from build123d import *

# Parameters (mm, degrees)
SKETCH1_W           = 51
SKETCH1_H           = 51
SKETCH1_R           = 1.5
BOSS_EXTRUDE1_DEPTH = 3


with BuildPart() as part:
    # Sketch1 → Boss-Extrude1 (new body)
    with BuildSketch(Plane(origin=(0, 0, 0), x_dir=(1, 0, 0), z_dir=(0, 1, 0))):
        Polygon((85, 1.25), (85, 3.5), (28, 3.5), (28, 28), (3.5, 28), (3.5, 85), (1.25, 85), (1.25, 100), (-1.25, 100), (-1.25, 85), (-3.5, 85), (-3.5, 28), (-28, 28), (-28, 3.5), (-85, 3.5), (-85, 1.25), (-100, 1.25), (-100, -1.25), (-85, -1.25), (-85, -3.5), (-28, -3.5), (-28, -28), (-3.5, -28), (-3.5, -85), (-1.25, -85), (-1.25, -100), (1.25, -100), (1.25, -85), (3.5, -85), (3.5, -28), (28, -28), (28, -3.5), (85, -3.5), (85, -1.25), (100, -1.25), (100, 1.25), align=None)
        Rectangle(SKETCH1_W, SKETCH1_H, mode=Mode.SUBTRACT)
        with Locations(Location((36, 0, 0), (0, 0, 270))):
            Circle(SKETCH1_R, mode=Mode.SUBTRACT)
        with Locations(Location((77, 0, 0), (0, 0, 270))):
            Circle(SKETCH1_R, mode=Mode.SUBTRACT)
        with Locations(Location((0, 77, 0), (0, 0, 270))):
            Circle(SKETCH1_R, mode=Mode.SUBTRACT)
        with Locations(Location((0, 36, 0), (0, 0, 270))):
            Circle(SKETCH1_R, mode=Mode.SUBTRACT)
        with Locations(Location((0, -36, 0), (0, 0, 270))):
            Circle(SKETCH1_R, mode=Mode.SUBTRACT)
        with Locations(Location((0, -77, 0), (0, 0, 270))):
            Circle(SKETCH1_R, mode=Mode.SUBTRACT)
        with Locations(Location((-36, 0, 0), (0, 0, 270))):
            Circle(SKETCH1_R, mode=Mode.SUBTRACT)
        with Locations(Location((-77, 0, 0), (0, 0, 270))):
            Circle(SKETCH1_R, mode=Mode.SUBTRACT)
    extrude(amount=BOSS_EXTRUDE1_DEPTH)


solid = part.part
Geometry: final body of the model. Coordinates: model frame, mm. Round coordinates to 2 decimals unless told otherwise and drop trailing zeros. Order: outer loops, then holes, each group sorted by start corner. A loop starts at its lowest first (then second) coordinate and runs counter-clockwise, first axis right, second up. Notation, with made-up numbers: (22.5, 8.5) -> (34.5, 8.5) arc R10 ccw to (34.5, 14.5) -> close; hole circle Ø2 at (-24.5, 60.5). An arc over 180 degrees is marked (long way). Put each result on its own line as item: value. Start each with the question number.
Q1. Section B-B on x = -49. Return the cut outline in (y, z).
Q2. Section A-A on x = -8. Return the cut outline in (y, z).
Q3. Section C-C on y = 1.85. Give the number of separate pieces and of enclosed holes in the cut face, and give its area (3 significant figures).
Q4. Line query: probe 1 along X at (y, z) = (1.7, 0); probe 2 along X at (y, z) = (1.9, -9.5); probe 3 along X at (y, z) = (1.5, 77). Output: solid intervals per line, ascending.
Q5. Section D-D on z = 32. Return the cut outline in (x, y), and give its area (3 significant figures).
Q6. First-contact query: pin 1 (2.5 mm diameter, centred on x = 0, z = -36, fed in from +Y); pin 2 (1 mm diameter, centred on x = -21, y = 2.5, fed in from +Z); pin 3 (1.1 mm diameter, centred on y = 2, z = -2.5, fed in from +X); pin 4 (1.5 mm diameter, centred on x = -59, y = 1, fed in from +Z). Flat tips, straight axial feed; report the tip coordinate or a pass-through.
Ans:
1. outline: (0, -3.5) -> (3, -3.5) -> (3, 3.5) -> (0, 3.5) -> close
2. outline: (0, -28) -> (3, -28) -> (3, -25.5) -> (0, -25.5) -> close; (0, 25.5) -> (3, 25.5) -> (3, 28) -> (0, 28) -> close
3. separate pieces: 1
3. enclosed holes: 9
3. area: 2,220 mm2
4. probe 1: x = -100 to -78.5, -75.5 to -37.5, -34.5 to -25.5, 25.5 to 34.5, 37.5 to 75.5, 78.5 to 100
4. probe 2: x = -28 to -25.5, 25.5 to 28
4. probe 3: x = -3.5 to -1.5, 1.5 to 3.5
5. outline: (-3.5, 0) -> (3.5, 0) -> (3.5, 3) -> (-3.5, 3) -> close
5. area: 21.0 mm2
6. pin 1: passes through
6. pin 2: stops at z = 28
6. pin 3: stops at x = 85
6. pin 4: stops at z = 3.5
